Could you check a few things on this model? Use its own coordinates, in mm. Face numbers are marked on the shaded views. A direction names the side the tool comes from. Coordinates: 2 decimals unless noted, no trailing zeros. Loops run counter-clockwise (first coordinate to the right, second up) from the corner with the lowest first, then second, coordinate; pieces in that order, holes last. Notation, with made-up numbers: (3.25, -13) -> (7.25, -13) arc R35 ccw to (7.25, 25) -> close; hole circle Ø3 at (-26, -17.75). An arc over 180 degrees is marked (long way). One line per question, with ' | ' between items.
from build123d import *

# Parameters (mm, degrees)
F0_W     = 42.3
F0_H     = 42.3
F1_DEPTH = 30
F2_SIZE  = 5
F5_R     = 1.25
F6_DEPTH = 5


with BuildPart() as f1:
    # F0 (on Top) → F1 (new body)
    with BuildSketch(Plane.XY):
        Rectangle(F0_W, F0_H)
    extrude(amount=F1_DEPTH)

    # F2
    f2_edges = [f1.edges().sort_by_distance(p)[0] for p in [
        (21.15, -21.15, 15),
        (-21.15, -21.15, 15),
        (-21.15, 21.15, 15),
        (21.15, 21.15, 15),
    ]]
    chamfer(f2_edges, length=F2_SIZE)

    # F3 (on Right) → F4 (revolve)
    with BuildSketch(Plane.YZ):
        Polygon((-11, 30), (0, 30), (0, 56), (-2.5, 56), (-2.5, 32), (-11, 32), align=None)
    revolve(axis=Axis((0, 0, 43), (0, 0, 1)))

    # F5 (on face) → F6 (cut)
    with BuildSketch(Plane.XY.offset(30)):
        with Locations((-15.5, 15.5)):
            Circle(F5_R)
        with Locations((15.5, 15.5)):
            Circle(F5_R)
        with Locations((15.5, -15.5)):
            Circle(F5_R)
        with Locations((-15.5, -15.5)):
            Circle(F5_R)
    extrude(amount=-F6_DEPTH, mode=Mode.SUBTRACT)


solid = f1.part
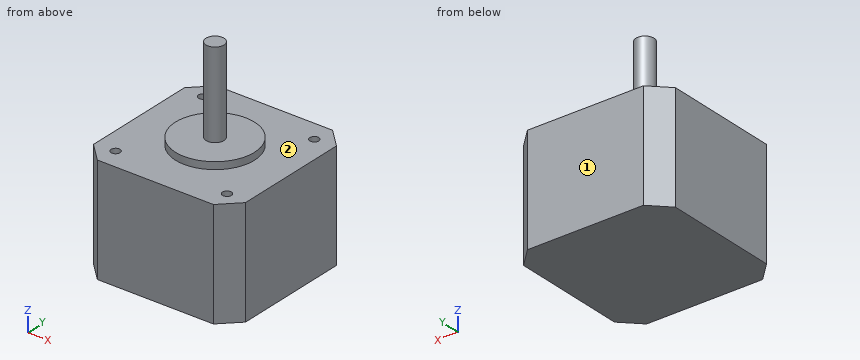
1) If we section it at A-A on z = 27: Please give me the cut outline in (x, y), and give its area (3 significant figures).
Data:
outline: (-21.15, -16.15) -> (-16.15, -21.15) -> (16.15, -21.15) -> (21.15, -16.15) -> (21.15, 16.15) -> (16.15, 21.15) -> (-16.15, 21.15) -> (-21.15, 16.15) -> close; hole circle Ø2.5 at (-15.5, -15.5); hole circle Ø2.5 at (-15.5, 15.5); hole circle Ø2.5 at (15.5, -15.5); hole circle Ø2.5 at (15.5, 15.5) | area: 1,720 mm²
2) On a 3-axis mill with a long thin cutter (end or side, diameter ignored), from which of +Z, -Z, +X, -X, +Y, -Y can I reach the whole of each face in a straight line? I mean the marked faces 1 and 2. Say none if no direction works.
Data:
face 1: +Z, -Z, +X, -X, +Y | face 2: +Z
3) If we section it at B-B on z = 11.5: Please give me the cut outline in (x, y).
Data:
outline: (-21.15, -16.15) -> (-16.15, -21.15) -> (16.15, -21.15) -> (21.15, -16.15) -> (21.15, 16.15) -> (16.15, 21.15) -> (-16.15, 21.15) -> (-21.15, 16.15) -> close
4) I need wall thicknesses on line 1 along Y through (x, z) = (15.5, 28.1); line 2 along Y through (x, z) = (-15, 28); line 3 along Z through (x, y) = (-10.5, -6.5). Which ranges of each line are inside material? Lowest first, please. Write a range as from..to.
Data:
line 1: -21.15..-16.75, -14.25..14.25, 16.75..21.15 | line 2: -21.15..-16.65, -14.35..14.35, 16.65..21.15 | line 3: 0..30
5) If we section it at C-C on x = 0: Please give me the cut outline in (y, z), and give its area (3 significant figures).
Data:
outline: (-21.15, 0) -> (21.15, 0) -> (21.15, 30) -> (11, 30) -> (11, 32) -> (2.5, 32) -> (2.5, 56) -> (-2.5, 56) -> (-2.5, 32) -> (-11, 32) -> (-11, 30) -> (-21.15, 30) -> close | area: 1,430 mm²
6) I'm going to push flat-ended pins straight in: pin 1 Ø3 at (x, y) = (15.5, 15) entering from +Z; pin 2 Ø11 at (x, y) = (-5.5, 2) entering from +Z; pin 3 Ø0.8 at (x, y) = (-16, -15.5) entering from +Z; pin 4 Ø1.5 at (x, y) = (-11.5, -1.5) entering from +Z. Where does each tip first touch, or does it pass through?
Data:
pin 1: z = 30 | pin 2: z = 56 | pin 3: z = 25 | pin 4: z = 32
